Read the model definition and answer for the solid it produces. Units are mm, in the model's axes. Face numbers are marked on the shaded views. A direction names the side the tool comes from. Give positions to 0.01 mm unless a question says otherwise; leave off trailing zeros. Order: outer loops, then holes, each group sorted by start corner. A loop starts at its lowest first (then second) coordinate and runs counter-clockwise, first axis right, second up. Notation, with made-up numbers: (8.5, 45) -> (63.5, 45) arc R10 ccw to (63.5, 60) -> close; hole circle Ø11 at (46, 85). An arc over 180 degrees is marked (long way). One line per question, with ' | ' between items. Start each with the question number.
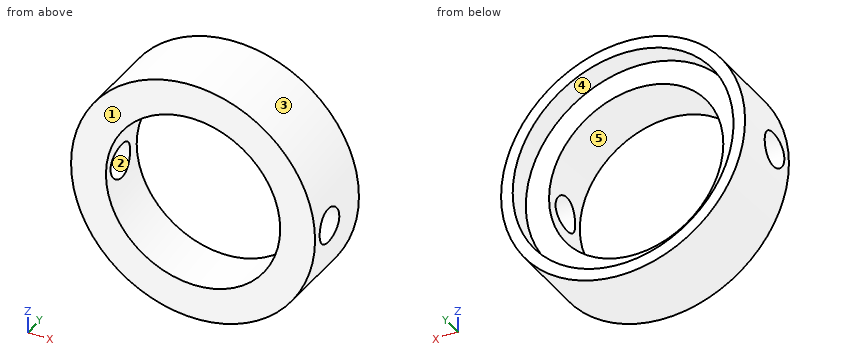
```python
from build123d import *

# Parameters (mm, degrees)
SCHIZZO1_R                    = 10.5
ESTRUSIONE_ESTRUSIONE1_DEPTH  = 7
SCHIZZO2_R                    = 9.5
TAGLIO_ESTRUSIONE1_DEPTH      = 2
SCHIZZO3_R                    = 7.5
TAGLIO_ESTRUSIONE2_DEPTH      = 6
SCHIZZO4_R                    = 1.5
TAGLIO_ESTRUSIONE3_DEPTH      = 11.5
TAGLIO_ESTRUSIONE3_DEPTH_BACK = 11.5
SCHIZZO6_R                    = 10.5
TAGLIO_ESTRUSIONE4_DEPTH      = 0.3


with BuildPart() as part:
    # Schizzo1 → Estrusione-Estrusione1 (new body)
    with BuildSketch(Plane(origin=(0, 0, 0), x_dir=(1, 0, 0), z_dir=(0, 1, 0))):
        Circle(SCHIZZO1_R)
    extrude(amount=ESTRUSIONE_ESTRUSIONE1_DEPTH)

    # Schizzo2 → Taglio-Estrusione1 (cut)
    with BuildSketch(Plane(origin=(0, 7, 0), x_dir=(1, 0, 0), z_dir=(0, 1, 0))):
        Circle(SCHIZZO2_R)
    extrude(amount=-TAGLIO_ESTRUSIONE1_DEPTH, mode=Mode.SUBTRACT)

    # Schizzo3 → Taglio-Estrusione2 (cut, through all)
    with BuildSketch(Plane(origin=(0, 5, 0), x_dir=(1, 0, 0), z_dir=(0, 1, 0))):
        Circle(SCHIZZO3_R)
    extrude(amount=-TAGLIO_ESTRUSIONE2_DEPTH, mode=Mode.SUBTRACT)

    # Schizzo4 → Taglio-Estrusione3 (cut, two sides)
    with BuildSketch(Plane(origin=(0, 0, 0), x_dir=(0, 0, -1), z_dir=(1, 0, 0))) as taglio_estrusione3_sk:
        with Locations((0, 2.5)):
            Circle(SCHIZZO4_R)
    extrude(amount=TAGLIO_ESTRUSIONE3_DEPTH, mode=Mode.SUBTRACT)
    extrude(taglio_estrusione3_sk.sketch, amount=-TAGLIO_ESTRUSIONE3_DEPTH_BACK, mode=Mode.SUBTRACT)

    # Schizzo6 → Taglio-Estrusione4 (cut)
    with BuildSketch(Plane.XZ):
        Circle(SCHIZZO6_R)
    extrude(amount=-TAGLIO_ESTRUSIONE4_DEPTH, mode=Mode.SUBTRACT)


solid = part.part
```
Q1. Given P1, Ø1.5, axis at y = 5, z = -1, coming from the +X side; P2, Ø3, axis at x = 7, y = 5.5, coming from the -Z side; P3, Ø2, axis at y = 4.5, z = -5.5, coming from the +X side, each flat-ended and moving along its own axis, determine where each tip first touches the part or whether it passes through.
Q2. A cutting plane is placed at B-B, the plane x = 0. Determine the outline of the cut face in (y, z).
Q3. A cutting plane is placed at D-D, the plane z = -3. Determine the outline of the cut face in (x, y), then the cut area to 3 significant figures.
Q4. Which of the six approach directions +Z, -Z, +X, -X, +Y, -Y give full straight-line access (tool end or side, diameter ignored) to the marked faces 4 and 5?
Q5. Determine the mould class of the marked faces 1, 2 and 3 for opening direction Z: pulls with the +Z half, pulls with the -Z half, needs draft (parallel to the pull), parting line crosses it, or undercut.
Q6. A cutting plane is placed at A-A, the plane z = 0. Determine the outline of the cut face in (x, y).
Q7. Find the intervals of material crossed by line 1 (Y direction, x = -8.3, z = 0); line 2 (Z direction, x = 0, y = 1.75); line 3 (X direction, y = 6.5, z = 0), in increasing order.
Geometry results:
1) P1: x = 10.5 | P2: z = -8.94 | P3: x = 9.49
2) outline: (0.3, -10.5) -> (7, -10.5) -> (7, -9.5) -> (5, -9.5) -> (5, -7.5) -> (0.3, -7.5) -> close; (0.3, 7.5) -> (5, 7.5) -> (5, 9.5) -> (7, 9.5) -> (7, 10.5) -> (0.3, 10.5) -> close
3) outline: (-10.06, 0.3) -> (-6.87, 0.3) -> (-6.87, 5) -> (-9.01, 5) -> (-9.01, 7) -> (-10.06, 7) -> close; (6.87, 0.3) -> (10.06, 0.3) -> (10.06, 7) -> (9.01, 7) -> (9.01, 5) -> (6.87, 5) -> close | area: 34.2 mm²
4) face 4: +Y | face 5: +Y, -Y
5) face 1: needs draft | face 2: undercut | face 3: parting line crosses it
6) outline: (-10.5, 0.3) -> (-7.5, 0.3) -> (-7.5, 1) -> (-10.5, 1) -> close; (-10.5, 4) -> (-7.5, 4) -> (-7.5, 5) -> (-9.5, 5) -> (-9.5, 7) -> (-10.5, 7) -> close; (7.5, 0.3) -> (10.5, 0.3) -> (10.5, 1) -> (7.5, 1) -> close; (7.5, 4) -> (10.5, 4) -> (10.5, 7) -> (9.5, 7) -> (9.5, 5) -> (7.5, 5) -> close
7) line 1: 0.3 to 1, 4 to 5 | line 2: -10.5 to -7.5, 7.5 to 10.5 | line 3: -10.5 to -9.5, 9.5 to 10.5
